Work out the finished part from the listing and answer in its coordinate system (mm). Face numbers are marked on the shaded views. A direction names the side the tool comes from. Give positions to 0.01 mm unless a question says otherwise; leave off trailing zeros. Loops run counter-clockwise (first coordinate to the right, second up) from the corner with the lowest first, then second, coordinate; pieces in that order, holes last. Notation, with made-up numbers: (34, 69.25) - (70, 69.25) arc R20 cw to (70, 76.25) - close; hole circle Ø7 at (-6.75, 62). An arc over 180 degrees is marked (long way). One line per question, with ' | ' between items. Start each with the question number.
1. Section A-A (x = 1.5) is taken. Determine the outline of the cut face in (y, z).
2. Find the intervals of material crossed by line 1 (Y direction, x = 2, z = -0.25); line 2 (Z direction, x = 1.5, y = 0); line 3 (Z direction, x = 1.9, y = 0), in increasing order.
3. Section C-C (x = 11) is taken. Determine the outline of the cut face in (y, z), plus the area to 3 significant figures.
4. For a pull along Y with two mould halves and no side action, classify the marked faces 3, 4 and 5 as released by +Y, released by -Y, zero draft, split by the parting line, or undercut.
5. Section B-B (x = 7.5) is taken. Determine the outline of the cut face in (y, z), plus the area to 3 significant figures.
6. Each of these flat-tipped pins is pushed along its axis until it touches: pin 1 (6 mm diameter, centred on y = 0, z = 0, fed in from -X); pin 2 (5 mm diameter, centred on y = 4.5, z = 6, fed in from +X); pin 3 (5 mm diameter, centred on x = 7, y = 1, fed in from +Z); pin 4 (6 mm diameter, centred on x = 3, y = -6.5, fed in from -Z). Where does it stop, or does it pass through?
7. Which of the six approach directions +Z, -Z, +X, -X, +Y, -Y give full straight-line access (tool end or side, diameter ignored) to the marked faces 1 and 2?
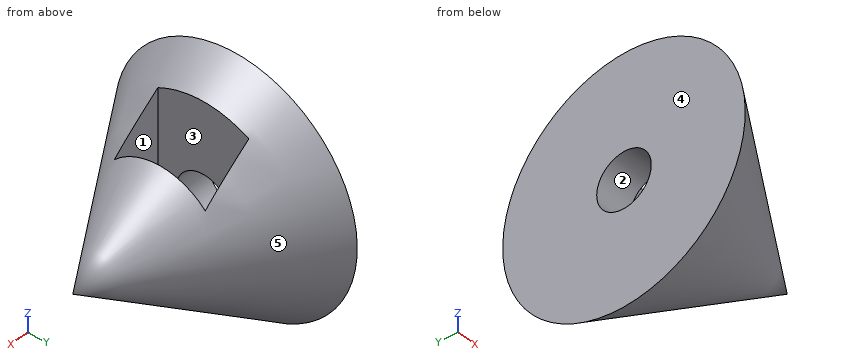
Autodesk Inventor part; units mm, degrees
ref_plane "Work Plane1" through (7, 0, 0) normal (1, 0, 0) x (0, 1, 0)
ref_plane "XZ Plane" through (0, 0, 0) normal (0, 1, 0) x (-1, 0, 0)
ref_plane "XY Plane" through (0, 0, 0) normal (0, 0, 1) x (1, 0, 0)
ref_plane "Work Plane1" through (7, 0, 0) normal (1, 0, 0) x (0, 1, 0)
sketch "Sketch1" plane through (0, 0, 0) normal (0, 1, 0) x (-1, 0, 0)
  line L0 (0, 0) -> (-15, 0)
  line L1 (0, 0) -> (0, -10)
  line L2 (-15, 0) -> (-15, 0)
  line L3 (-15, 0) -> (0, -10)
  dimension "d0" = 15
  dimension "d1" = 10
  dimension "d2" = 0
revolve "Revolution1" add sketch "Sketch1" angle 360 about axis through (0, 0, 0) along (1, 0, 0)
sketch "Sketch2" plane through (7, 0, 0) normal (1, 0, 0) x (0, 1, 0)
  circle A0 centre (0, 0) radius 2.25
  dimension "d5" = 4.5
extrude "Extrusion1" cut sketch "Sketch2" along normal blind 2 and the other way blind 10
sketch "Sketch3" plane through (7, 0, 0) normal (1, 0, 0) x (0, 1, 0)
  line L0 (0, 0) -> (3.75, 0)
  line L1 (3.75, -2.1651) -> (0, -4.3301)
  line L2 (0, -4.3301) -> (-3.75, -2.1651)
  line L3 (-3.75, -2.1651) -> (-3.75, 2.1651)
  line L4 (-3.75, 2.1651) -> (0, 4.3301)
  line L5 (0, 4.3301) -> (3.75, 2.1651)
  line L6 (3.75, 2.1651) -> (3.75, -2.1651)
  line L7 (-3.75, 14.6203) -> (-3.75, 2.1651)
  line L8 (-3.75, 14.6203) -> (3.75, 14.6203)
  line L9 (3.75, 14.6203) -> (3.75, 1.2022)
  line L10 (3.75, 1.2022) -> (-3.75, 1.2022)
  line L11 (-3.75, 1.2022) -> (-3.75, 14.6203)
  dimension "d15" = 3.75
extrude "Extrusion2" cut sketch "Sketch3" against normal blind 4
sketch "Sketch5" plane through (9, 0, 0) normal (-1, 0, 0) x (0, 0, 1)
  circle A0 centre (0, 0) radius 2.25
extrude "Extrusion3" add sketch "Sketch5" along normal up to surface (2 mm away)
properties part number "stollen_m4_spitz"
Conclusion:
1) outline: circle Ø18 at (0, 0); hole circle Ø4.5 at (0, 0)
2) line 1: -8.66 to -2.24, 2.24 to 8.66 | line 2: -9 to -2.25, 2.25 to 9 | line 3: -8.73 to -2.25, 2.25 to 8.73
3) outline: circle Ø5.33 at (0, 0) | area: 22.3 mm²
4) face 3: undercut | face 4: zero draft | face 5: split by the parting line
5) outline: circle Ø10 at (0, 0) | area: 78.5 mm²
6) pin 1: x = 0 | pin 2: x = 7.5 | pin 3: z = 5.33 | pin 4: z = -8.37
7) face 1: +Z | face 2: -X
